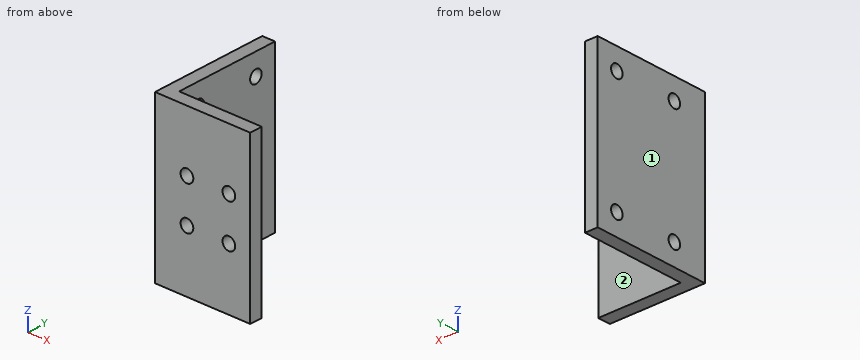
from build123d import *

# Parameters (mm, degrees)
SKETCH_1_W          = 22.5
SKETCH_1_H          = 38
EXTRUDE_1_DEPTH     = 3
SKETCH_2_W          = 3
SKETCH_2_H          = 38
EXTRUDE_2_DEPTH     = 25
SKETCH_3_R          = 1.5
CUT_EXTRUDE_2_DEPTH = 25
SKETCH_4_R          = 1.5
CUT_EXTRUDE_3_DEPTH = 25


with BuildPart() as part:
    # 草图1 → 凸台-拉伸1 (new body)
    with BuildSketch(Plane(origin=(0, 0, 0), x_dir=(1, 0, 0), z_dir=(0, 1, 0))):
        Rectangle(SKETCH_1_W, SKETCH_1_H)
    extrude(amount=EXTRUDE_1_DEPTH)

    # 草图2 → 凸台-拉伸2 (add)
    with BuildSketch(Plane(origin=(0, 3, 0), x_dir=(1, 0, 0), z_dir=(0, 1, 0))):
        with Locations((-9.75, 0)):
            Rectangle(SKETCH_2_W, SKETCH_2_H)
    extrude(amount=EXTRUDE_2_DEPTH)

    # 草图3 → 切除-拉伸2 (cut)
    with BuildSketch(Plane.XZ):
        with Locations(Location((-3.699747468, 5.049747468, 0), (0, 0, 270))):
            Circle(SKETCH_3_R)
        with Locations(Location((6.199747468, 5.049747468, 0), (0, 0, 270))):
            Circle(SKETCH_3_R)
        with Locations(Location((-3.699747468, -4.849747468, 0), (0, 0, 270))):
            Circle(SKETCH_3_R)
        with Locations(Location((6.199747468, -4.849747468, 0), (0, 0, 270))):
            Circle(SKETCH_3_R)
    extrude(amount=-CUT_EXTRUDE_2_DEPTH, mode=Mode.SUBTRACT)

    # 草图4 → 切除-拉伸3 (cut)
    with BuildSketch(Plane(origin=(-8.25, 0, 0), x_dir=(0, 0, -1), z_dir=(1, 0, 0))):
        with Locations((14, 23)):
            Circle(SKETCH_4_R)
        with Locations((-14, 23)):
            Circle(SKETCH_4_R)
        with Locations((-14, 8)):
            Circle(SKETCH_4_R)
        with Locations((14, 8)):
            Circle(SKETCH_4_R)
    extrude(amount=-CUT_EXTRUDE_3_DEPTH, mode=Mode.SUBTRACT)


solid = part.part
Can you work these out from the model? Positions are in its coordinate system, mm. Face numbers are marked on the shaded views. A direction names the side the tool comes from. Coordinates: 2 decimals unless noted, no trailing zeros. Loops run counter-clockwise (first coordinate to the right, second up) from the corner with the lowest first, then second, coordinate; pieces in that order, holes last. Notation, with made-up numbers: (-24, -9) - (-5, -9) arc R32 cw to (-5, 22) - close; hole circle Ø11 at (63.5, 66.25). An arc over 180 degrees is marked (long way). Answer as a JSON object with one key per item and string values. Group by question number.
Item 1: If we section it at B-B (z = -14): List the corners of the cut face in (x, y) for me.
Item 2: If we section it at A-A (y = 8): List the corners of the cut face in (x, z) for me.
Item 3: If we section it at D-D (z = -2.5): List the corners of the cut face in (x, y) for me, plus the area to 4 significant figures.
Item 4: On a 3-axis mill with a long thin cutter (end or side, diameter ignored), from which of +Z, -Z, +X, -X, +Y, -Y can I reach the whole of each face in a straight line? I mean the marked faces 1 and 2. Say none if no direction works.
Item 5: If we section it at C-C (x = 5.75): List the corners of the cut face in (y, z) for me, plus the area to 3 significant figures.
Item 6: If I drill on L1, parallel to Y at x = -9.2, z = 14; L2, parallel to X at y = 2, z = 5.5; L3, parallel to Z at x = -8.75, y = 8.75, over which ranges is the centre line in solid material (lowest first)? Write a range as from..to.
Item 7: For pin 1 (1.5 mm diameter, centred on y = 15, z = 9, fed in from +X); pin 2 (1 mm diameter, centred on x = -3, z = 1, fed in from +Y), each with a flat end and sliding along its axis, tell me the tip position at first contact or that it passes through.
Returned:
{
 "1": {"outline": "(-11.25, 0) - (11.25, 0) - (11.25, 3) - (-8.25, 3) - (-8.25, 6.5) - (-11.25, 6.5) - close; (-11.25, 9.5) - (-8.25, 9.5) - (-8.25, 21.5) - (-11.25, 21.5) - close; (-11.25, 24.5) - (-8.25, 24.5) - (-8.25, 28) - (-11.25, 28) - close"},
 "2": {"outline": "(-11.25, -19) - (-8.25, -19) - (-8.25, -15.5) - (-11.25, -15.5) - close; (-11.25, -12.5) - (-8.25, -12.5) - (-8.25, 12.5) - (-11.25, 12.5) - close; (-11.25, 15.5) - (-8.25, 15.5) - (-8.25, 19) - (-11.25, 19) - close"},
 "3": {"outline": "(-11.25, 0) - (11.25, 0) - (11.25, 3) - (-8.25, 3) - (-8.25, 28) - (-11.25, 28) - close", "area": "142.5 mm²"},
 "4": {"face 1": "+Z, -Z, -X, +Y, -Y", "face 2": "+Z, -Z, +X, +Y"},
 "5": {"outline": "(0, -19) - (3, -19) - (3, -6.28) - (0, -6.28) - close; (0, -3.42) - (3, -3.42) - (3, 3.62) - (0, 3.62) - close; (0, 6.48) - (3, 6.48) - (3, 19) - (0, 19) - close", "area": "96.8 mm²"},
 "6": {"L1": "y = 0..6.5, 9.5..21.5, 24.5..28", "L2": "x = -11.25..-5.13, -2.27..4.77, 7.63..11.25", "L3": "z = -19..-15.3, -12.7..12.7, 15.3..19"},
 "7": {"pin 1": "stops at x = -8.25", "pin 2": "stops at y = 3"}
}
